Check sheet for the drawn part. Datum: minimum x, y, z corner. Units: mm. Coordinates: 2 decimals unless noted, no trailing zeros. Loops run counter-clockwise (first coordinate to the right, second up) from the corner with the lowest first, then second, coordinate; pieces in that order, holes last. Notation, with made-up numbers: (-16, 12.5) -> (-7, 12.5) arc R24 ccw to (-7, 51.5) -> close; hole circle Ø8 at (65.25, 60). An arc over 180 degrees is marked (long way). Use CSV: the item, a comma, the result in double quotes. Start each with the question number.
1. Sectioned sample at A-A, the plane x = 22.5. Record the cut outline in (y, z).
2. Gauge pin test, flat ends, axial feed: pin 1 (1.2 mm diameter, centred on x = 67, z = 12, fed in from +Y); pin 2 (1.2 mm diameter, centred on y = 39.5, z = 11.5, fed in from +X); pin 3 (4.5 mm diameter, centred on y = 40.5, z = 11, fed in from +X); pin 4 (24 mm diameter, centred on x = 60, y = 58, fed in from +Z). Record the tip position at first contact, or that the pin passes through.
3. Thickness scan on L1, parallel to Z at x = 11.5, y = 57; L2, parallel to Y at x = 67.5, z = 13. Record the ranges inside material, lowest first.
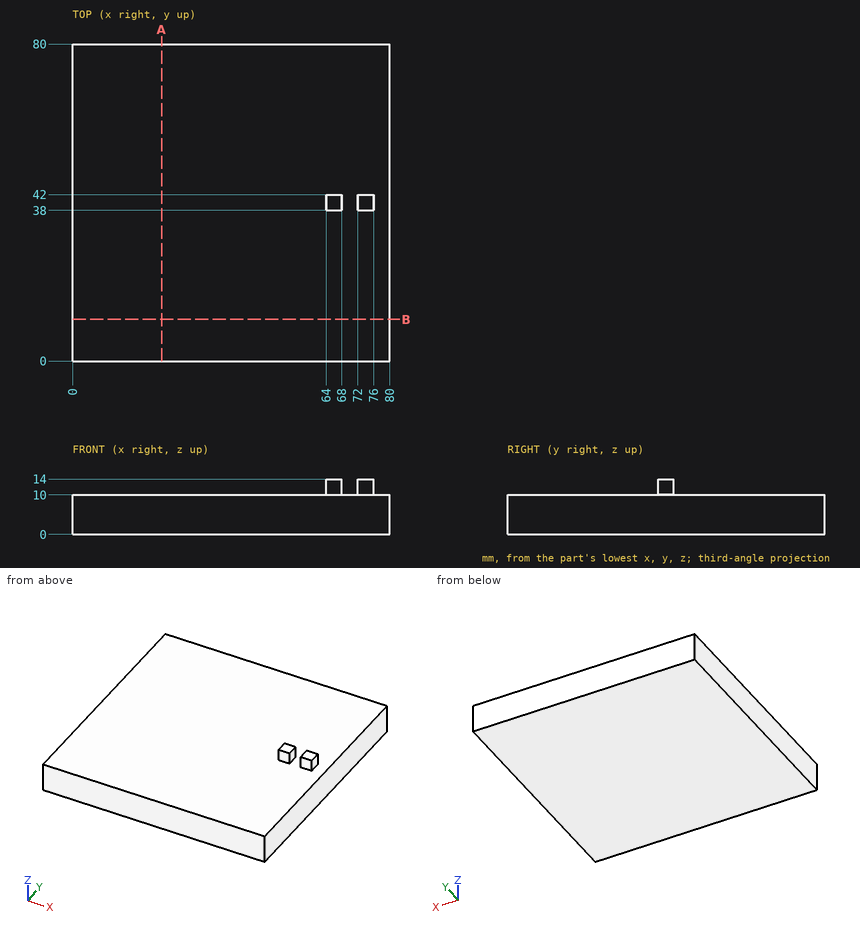
Completed:
1,outline,"(0, 0) -> (80, 0) -> (80, 10) -> (0, 10) -> close"
2,pin 1,"y = 42"
2,pin 2,"x = 76"
2,pin 3,"x = 80"
2,pin 4,"z = 10"
3,L1,"0 to 10"
3,L2,"38 to 42"
